Input: part model. Units: mm. Frame: model coordinates. A direction names the side the tool comes from. Coordinates: 2 decimals unless noted, no trailing zeros. Loops run counter-clockwise (first coordinate to the right, second up) from the corner with the lowest first, then second, coordinate; pieces in that order, holes last.
```python
from build123d import *

# Parameters (mm, degrees)
SKETCH1_W           = 14.5
SKETCH1_H           = 13
SKETCH1_W_2         = 9
SKETCH1_H_2         = 9
BOSS_EXTRUDE1_DEPTH = 1.5
SKETCH2_W           = 1.5
SKETCH2_H           = 13
BOSS_EXTRUDE2_DEPTH = 25
SKETCH3_W           = 1.5
SKETCH3_H           = 13
BOSS_EXTRUDE3_DEPTH = 1.5


with BuildPart() as part:
    # Sketch1 → Boss-Extrude1 (new body)
    with BuildSketch(Plane.XY):
        Rectangle(SKETCH1_W, SKETCH1_H)
        with Locations((0.75, 0)):
            Rectangle(SKETCH1_W_2, SKETCH1_H_2, mode=Mode.SUBTRACT)
    extrude(amount=BOSS_EXTRUDE1_DEPTH)

    # Sketch2 → Boss-Extrude2 (add)
    with BuildSketch(Plane(origin=(0, 0, 0), x_dir=(-1, 0, 0), z_dir=(0, 0, -1))):
        with Locations((6.5, 0)):
            Rectangle(SKETCH2_W, SKETCH2_H)
    extrude(amount=BOSS_EXTRUDE2_DEPTH)

    # Sketch3 → Boss-Extrude3 (add)
    with BuildSketch(Plane(origin=(-5.75, 0, 0), x_dir=(0, 0, -1), z_dir=(1, 0, 0))):
        with Locations((24.25, 0)):
            Rectangle(SKETCH3_W, SKETCH3_H)
    extrude(amount=BOSS_EXTRUDE3_DEPTH)


solid = part.part
```
Item 1: Line query: L1, parallel to Z at x = -4.75, y = 2.5; L2, parallel to X at y = 3.75, z = -15; L3, parallel to Z at x = 5.5, y = 0. Output: solid intervals per line, ascending.
Result:
L1: z = -25 to -23.5, 0 to 1.5
L2: x = -7.25 to -5.75
L3: z = 0 to 1.5
Item 2: Section query A-A (y = 0.25). Output: boundary loops of the cut face in (x, z).
Result:
outline: (-7.25, -25) - (-4.25, -25) - (-4.25, -23.5) - (-5.75, -23.5) - (-5.75, 0) - (-3.75, 0) - (-3.75, 1.5) - (-7.25, 1.5) - close; (5.25, 0) - (7.25, 0) - (7.25, 1.5) - (5.25, 1.5) - close
Item 3: Section query B-B (x = 0.5). Output: boundary loops of the cut face in (y, z).
Result:
outline: (-6.5, 0) - (-4.5, 0) - (-4.5, 1.5) - (-6.5, 1.5) - close; (4.5, 0) - (6.5, 0) - (6.5, 1.5) - (4.5, 1.5) - close
Item 4: Mould query, pull axis Y, two halves, no side actions, for faces 4 (the face through (1, 4.5, 1)), 5 (the face through (-6, -6.5, -8)), 6 (the face through (-5.75, 0, -12)), 7 (the face through (1, -4.5, 1)). Classes: +Y half, -Y half, draft (parallel to the pull), parting line (faces both ways), or undercut.
Result:
face 4: undercut
face 5: -Y half
face 6: draft
face 7: undercut
Item 5: Section query C-C (z = -17). Output: boundary loops of the cut face in (x, y).
Result:
outline: (-7.25, -6.5) - (-5.75, -6.5) - (-5.75, 6.5) - (-7.25, 6.5) - close
Item 6: Contact query for a flat-ended pin moving along its axis: P1, Ø1.5, axis at y = 4, z = -17, coming from the +X side. Output: stop coordinate, or through.
Result:
P1: stops at x = -5.75
Item 7: Reachability of faces 1 (the face through (-4.25, 0, -24)), 2 (the face through (5.25, 0, 1)), 3 (the face through (-5, 0, -23.5)) from +Z, -Z, +X, -X, +Y, -Y: full face, straight path, thin tool, end or side. Return the list, or none.
Result:
face 1: -Z, +X, +Y, -Y
face 2: +Z, -Z
face 3: +X, +Y, -Y
